For this review, take the finished solid that the model builds, in its own axes (mm). Give positions to 0.01 mm unless a question says otherwise; leave off trailing zeros. Write each loop counter-clockwise with the first axis right and the second up, starting at its lowest first coordinate (ties: lowest second). Pieces come first, ordered by that corner, then holes. Notation, with made-up numbers: M 4,-36 L 18,-36 A24 ccw 18,3 Z; hole C -40,64 d3. An arc over 180 degrees is marked long. Use one line per item in the form item = value. Start each with the question number.
Q1. Clearance check with flat-ended pins moving along their axes: pin 1 Ø4 at (x, y) = (-15, 53) entering from +Z; pin 2 Ø4 at (x, y) = (-8.5, 108.5) entering from -Z; pin 3 Ø6.5 at (y, z) = (64, 9.5) entering from +X; pin 4 Ø6.5 at (y, z) = (159.5, 8.5) entering from -X. State where each tip first meets the part, or that it passes through.
Q2. For probe 1 along X at (y, z) = (127, 17.75); probe 2 along Z at (x, y) = (-3.5, 27); probe 3 along Z at (x, y) = (-7, 72.5), list the stretches that pass through material, from the lowest coordinate up. Write a range as [from, to].
Q3. Consider section C-C on x = -11. Write out the cut boundary in (y, z).
Q4. Consider section B-B on z = 10. Write out the cut boundary in (x, y), and give its area (3 significant figures).
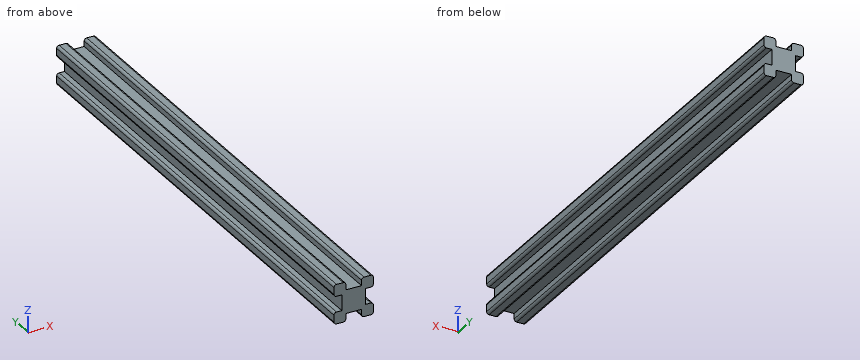
Autodesk Inventor part; units mm, degrees
ref_plane "Work Plane1" through (-4.73, 0, 10) normal (0, 0, 1) x (1, 0, 0)
ref_plane "YZ Plane" through (0, 0, 0) normal (1, 0, 0) x (0, 1, 0)
ref_plane "XZ Plane" through (0, 0, 0) normal (0, 1, 0) x (-1, 0, 0)
sketch "Sketch1" plane through (0, 0, 0) normal (0, 1, 0) x (-1, 0, 0)
  line L0 (0, 0) -> (20, 0)
  line L1 (20, 0) -> (20, 20)
  line L2 (20, 20) -> (0, 20)
  line L3 (0, 20) -> (0, 0)
  line L4 (6, 0) -> (14, 0)
  line L5 (14, 0) -> (14, 4)
  line L6 (14, 4) -> (6, 4)
  line L7 (6, 4) -> (6, 0)
  line L8 (0, 6) -> (4, 6)
  line L9 (4, 6) -> (4, 14)
  line L10 (4, 14) -> (0, 14)
  line L11 (0, 14) -> (0, 6)
  line L12 (6, 20) -> (14, 20)
  line L13 (14, 20) -> (14, 16)
  line L14 (14, 16) -> (6, 16)
  line L15 (6, 16) -> (6, 20)
  line L16 (20, 14) -> (16, 14)
  line L17 (16, 14) -> (16, 6)
  line L18 (16, 6) -> (20, 6)
  line L19 (20, 6) -> (20, 14)
  dimension "d0" = 20
  dimension "d1" = 20
  dimension "d2" = 8
  dimension "d3" = 6
  dimension "d4" = 8
  dimension "d5" = 6
  dimension "d6" = 4
  dimension "d7" = 4
  dimension "d8" = 4
  dimension "d9" = 4
extrude "Extrusion1" add sketch "Sketch1" along normal blind 254 contours L3 L8 L9 L10 L2 L15 L14 L13 L1 L16 L17 L18 L0 L5 L6 L7
fillet "Fillet1" radius 1.27 12 edges at (0, 127, 20) (0, 127, 14) (-6, 127, 20) (-14, 127, 20) (-20, 127, 20) (-20, 127, 14) (0, 127, 6) (0, 127, 0) (-6, 127, 0) (-14, 127, 0) (-20, 127, 0) (-20, 127, 6)
ref_plane "Work Plane1" through (-4.73, 0, 10) normal (0, 0, 1) x (1, 0, 0)
properties part number "20x20extrusionshort" material "Aluminum 6061"
Working result:
q1.pin_1 = 20
q1.pin_2 = 4
q1.pin_3 = -4
q1.pin_4 = -19.89
q2.probe_1 = [-20, -14], [-6, 0]
q2.probe_2 = [0, 6], [14, 20]
q2.probe_3 = [4, 16]
q3.outline = M 0,4 L 254,4 L 254,16 L 0,16 Z
q4.outline = M -16,0 L -4,0 L -4,254 L -16,254 Z
q4.area = 3,050 mm²
